Geometry check sheet. Reference: drawing and pictorial views, mm from the part's lowest x, y, z. A direction names the side the tool comes from. Round coordinates to 2 decimals unless told otherwise and drop trailing zeros. Write each loop counter-clockwise with the first axis right and the second up, starting at its lowest first coordinate (ties: lowest second). Pieces come first, ordered by that corner, then holes. Notation, with made-up numbers: (-25, 86) - (24, 86) arc R22 ccw to (24, 115) - close; hole circle Ø6 at (-21, -38.5). An arc over 180 degrees is marked (long way). Return JSON: item names as keys, results as strings.
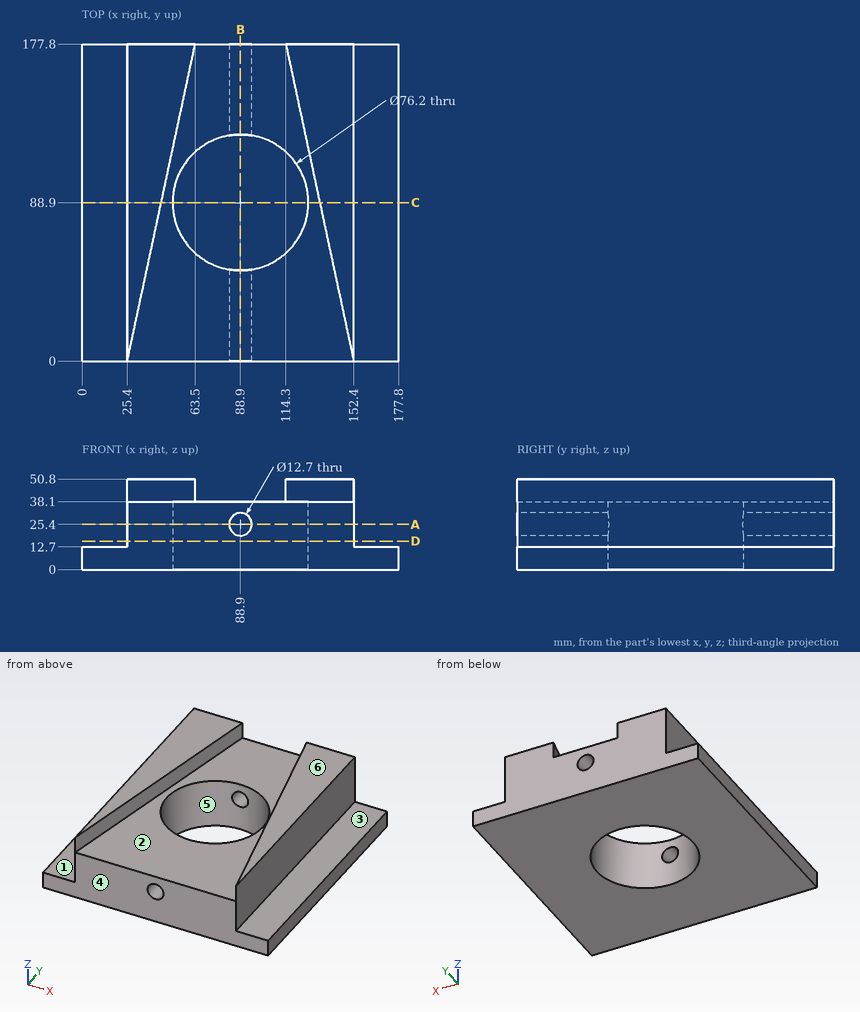
(1) Section check B-B, the plane x = 88.9. Enter the section's corners in (y, z).
Response values:
{"outline": "(0, 0) - (50.8, 0) - (50.8, 19.05) - (0, 19.05) - close; (0, 31.75) - (50.8, 31.75) - (50.8, 38.1) - (0, 38.1) - close; (127, 0) - (177.8, 0) - (177.8, 19.05) - (127, 19.05) - close; (127, 31.75) - (177.8, 31.75) - (177.8, 38.1) - (127, 38.1) - close"}
(2) Release check for a two-part mould opening along Y. For the marked faces 4, 5 and 6 record: pulls with the +Y half, pulls with the -Y half, needs draft (parallel to the pull), parting line crosses it, or undercut.
Response values:
{"face 4": "pulls with the -Y half", "face 5": "undercut", "face 6": "needs draft"}
(3) Access from +Z, -Z, +X, -X, +Y, -Y to the whole of each face (thin tool, end or side, straight path). Record for the marked faces 1, 2 and 3.
Response values:
{"face 1": "+Z, -X, +Y, -Y", "face 2": "+Z, -Y", "face 3": "+Z, +X, +Y, -Y"}
(4) Section check C-C, the plane y = 88.9. Enter the section's corners in (x, z).
Response values:
{"outline": "(0, 0) - (50.8, 0) - (50.8, 38.1) - (44.45, 38.1) - (44.45, 50.8) - (25.4, 50.8) - (25.4, 12.7) - (0, 12.7) - close; (127, 0) - (177.8, 0) - (177.8, 12.7) - (152.4, 12.7) - (152.4, 50.8) - (133.35, 50.8) - (133.35, 38.1) - (127, 38.1) - close"}
(5) Material ranges on line 1 along Z through (x, y) = (88.9, 163); line 2 along X through (y, z) = (88, 15); line 3 along X through (y, z) = (45, 24.5), recorded low to high. Write a range as [from, to].
Response values:
{"line 1": "z = [0, 19.05], [31.75, 38.1]", "line 2": "x = [25.4, 50.81], [126.99, 152.4]", "line 3": "x = [25.4, 82.61], [95.19, 152.4]"}
(6) Gauge pin test, flat ends, axial feed: pin 1 (8 mm diameter, centred on y = 63, z = 17.5, fed in from +X); pin 2 (10 mm diameter, centred on x = 88.9, z = 25.4, fed in from +Y); pin 3 (6 mm diameter, centred on y = 146, z = 32.5, fed in from -X); pin 4 (7.5 mm diameter, centred on x = 163, y = 93.5, fed in from +Z). Record the tip position at first contact, or that the pin passes through.
Response values:
{"pin 1": "stops at x = 152.4", "pin 2": "passes through", "pin 3": "stops at x = 25.4", "pin 4": "stops at z = 12.7"}
(7) Section check D-D, the plane z = 16. Enter the section's corners in (x, y).
Response values:
{"outline": "(25.4, 0) - (152.4, 0) - (152.4, 177.8) - (25.4, 177.8) - close; hole circle Ø76.2 at (88.9, 88.9)"}
(8) Section check A-A, the plane z = 25.4. Enter the section's corners in (x, y), plus the area to 3 significant figures.
Response values:
{"outline": "(25.4, 0) - (82.55, 0) - (82.55, 51.33) arc R38.1 cw to (82.55, 126.47) - (82.55, 177.8) - (25.4, 177.8) - close; (95.25, 0) - (152.4, 0) - (152.4, 177.8) - (95.25, 177.8) - (95.25, 126.47) arc R38.1 cw to (95.25, 51.33) - close", "area": "16,700 mm^2"}
